Geometry check sheet. Reference: drawing and pictorial views, mm from the part's lowest x, y, z. Give positions to 0.01 mm unless a question says otherwise; leave off trailing zeros. Write each loop counter-clockwise with the first axis right and the second up, starting at its lowest first coordinate (ties: lowest second). Pieces come first, ordered by that corner, then holes. Notation, with made-up numbers: (12, -24.75) -> (68, -24.75) arc R19 ccw to (68, 8.25) -> close; hole circle Ø4 at (-6, 81.5). An arc over 180 degrees is marked (long way). Use a Markdown table: item, result. Add a question column.
1. Scan lines: probe 1 along X at (y, z) = (90.5, 38); probe 2 along X at (y, z) = (122, 9.5); probe 3 along X at (y, z) = (82, 19). Record each from-to range of solid material in increasing order. Write a range as [from, to].
2. Cross-section at B-B (z = 31). Enter the section's corners in (x, y).
3. Cross-section at D-D (z = 21). Enter the section's corners in (x, y).
4. Cross-section at C-C (z = 9). Enter the section's corners in (x, y), then the cut area to 3 significant figures.
5. Gauge pin test, flat ends, axial feed: P1, Ø1.6, axis at x = 5.5, y = 64, coming from the +Z side; P2, Ø1, axis at y = 122.5, z = 29.5, coming from the -X side; P3, Ø10, axis at y = 52.5, z = 29, coming from the -X side. Record the tip position at first contact, or that the pin passes through.
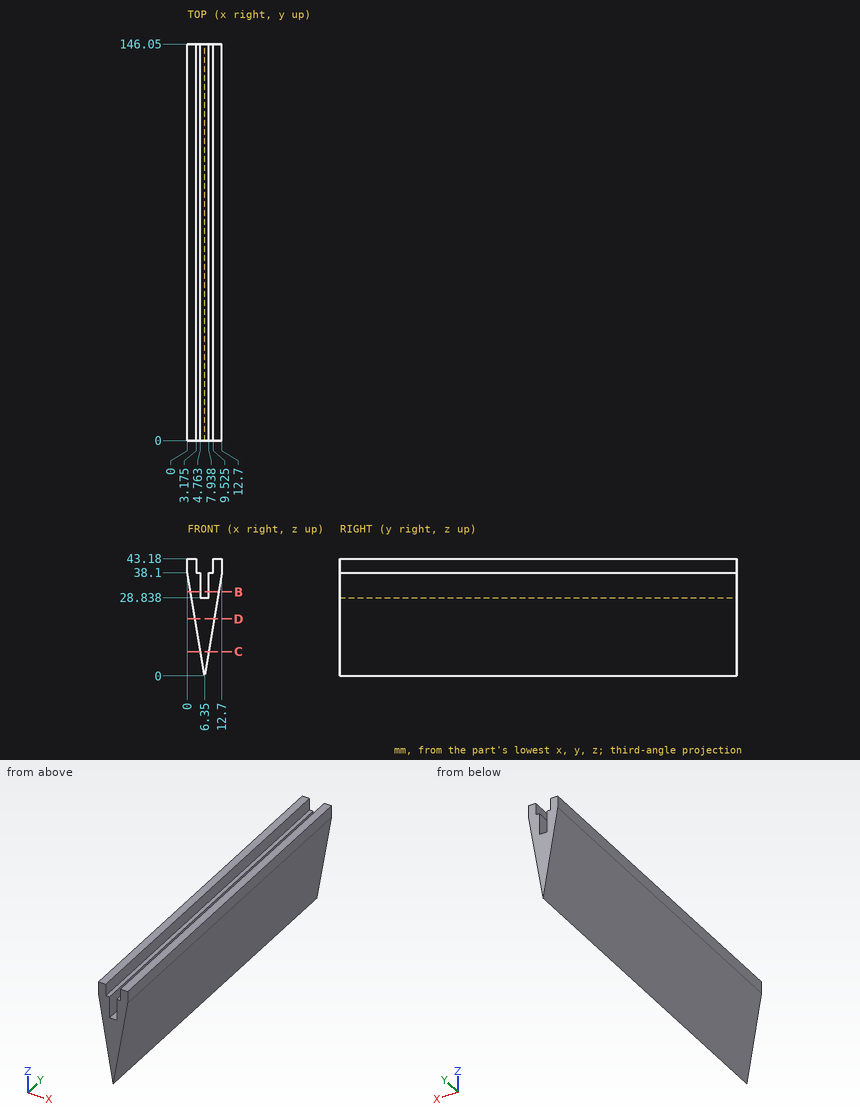
Worked answers:
| question | item | result |
|---|---|---|
| 1 | probe 1 | x = [0.02, 4.76], [7.94, 12.68] |
| 1 | probe 2 | x = [4.77, 7.93] |
| 1 | probe 3 | x = [3.18, 9.52] |
| 2 | outline | (1.18, 0) -> (4.76, 0) -> (4.76, 146.05) -> (1.18, 146.05) -> close; (7.94, 0) -> (11.52, 0) -> (11.52, 146.05) -> (7.94, 146.05) -> close |
| 3 | outline | (2.85, 0) -> (9.85, 0) -> (9.85, 146.05) -> (2.85, 146.05) -> close |
| 4 | outline | (4.85, 0) -> (7.85, 0) -> (7.85, 146.05) -> (4.85, 146.05) -> close |
| 4 | area | 438 mm² |
| 5 | P1 | stops at z = 38.1 |
| 5 | P2 | stops at x = 1.35 |
| 5 | P3 | stops at x = 0.68 |
